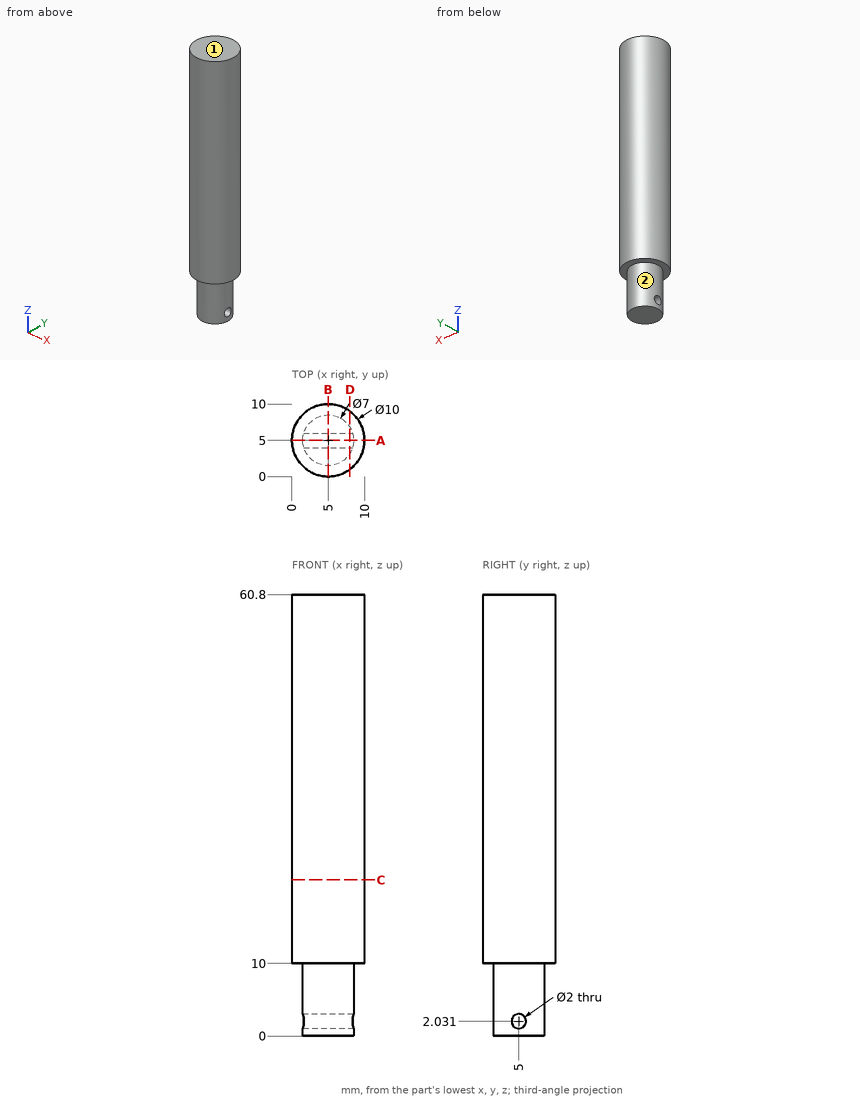
Input: dimensioned drawing with shaded views. Units: mm. Origin: part minimum x, y, z. A direction names the side the tool comes from. Coordinates: 2 decimals unless noted, no trailing zeros. Loops run counter-clockwise (first coordinate to the right, second up) from the corner with the lowest first, then second, coordinate; pieces in that order, holes last. Notation, with made-up numbers: (-24, 85) - (24, 85) arc R7 cw to (24, 91) - close; hole circle Ø5 at (-6, 9). An arc over 180 degrees is marked (long way). One line per question, with ' | ' between items. Start each with the question number.
(1) Cut plane B-B on x = 5. Output: boundary loops of the cut face in (y, z), and give its area (3 significant figures).
(2) Cut plane D-D on x = 8. Output: boundary loops of the cut face in (y, z), and give its area (3 significant figures).
(3) Cut plane A-A on y = 5. Output: boundary loops of the cut face in (x, z).
(4) First-contact query: pin 1 (1.6 mm diameter, centred on y = 5, z = 2.03, fed in from +X); pin 2 (4 mm diameter, centred on x = 2.5, z = 7.5, fed in from +Y); pin 3 (3 mm diameter, centred on y = 8.5, z = 46.5, fed in from +X). Flat tips, straight axial feed; report the tip coordinate or a pass-through.
(5) Ray query, L1, parallel to Z at x = 5.5, y = 5; L2, parallel to Z at x = 1.5, y = 7.5; L3, parallel to Y at x = 5.25, z = 29. Return the intervals inside material, ascending. Write a range as from..to.
(6) Cut plane C-C on z = 21.5. Output: boundary loops of the cut face in (x, y).
(7) Reachability of the marked faces 1 and 2 from +Z, -Z, +X, -X, +Y, -Y: full face, straight path, thin tool, end or side. Return the list, or none.
Here are the results:
1) outline: (0, 10) - (1.5, 10) - (1.5, 0) - (8.5, 0) - (8.5, 10) - (10, 10) - (10, 60.8) - (0, 60.8) - close; hole circle Ø2 at (5, 2.03) | area: 575 mm²
2) outline: (1, 10) - (3.2, 10) - (3.2, 0) - (6.8, 0) - (6.8, 10) - (9, 10) - (9, 60.8) - (1, 60.8) - close; hole circle Ø2 at (5, 2.03) | area: 439 mm²
3) outline: (0, 10) - (1.5, 10) - (1.5, 3.03) - (8.5, 3.03) - (8.5, 10) - (10, 10) - (10, 60.8) - (0, 60.8) - close; (1.5, 0) - (8.5, 0) - (8.5, 1.03) - (1.5, 1.03) - close
4) pin 1: through | pin 2: y = 8.46 | pin 3: x = 9.58
5) L1: 0..1.03, 3.03..60.8 | L2: 10..60.8 | L3: 0.01..9.99
6) outline: circle Ø10 at (5, 5)
7) face 1: +Z, +X, -X, +Y, -Y | face 2: -Z
